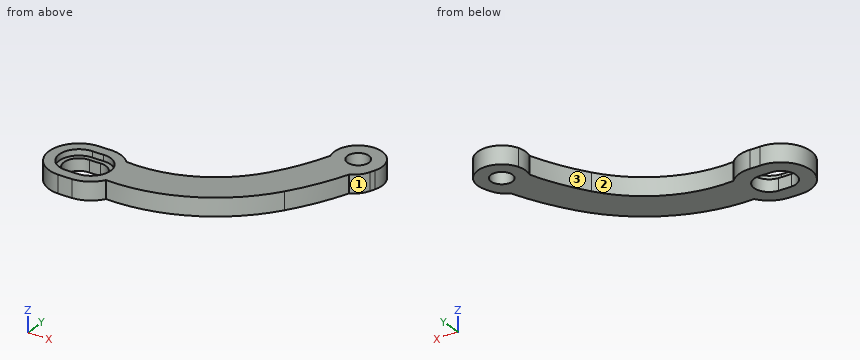
Autodesk Inventor part; units mm, degrees
ref_plane "YZ Plane" through (0, 0, 0) normal (1, 0, 0) x (0, 1, 0)
ref_plane "XZ Plane" through (0, 0, 0) normal (0, 1, 0) x (-1, 0, 0)
ref_plane "XY Plane" through (0, 0, 0) normal (0, 0, 1) x (1, 0, 0)
sketch "Sketch1" plane through (0, 0, 0) normal (0, 0, 1) x (1, 0, 0)
  circle A0 centre (31, 22) radius 1.25
  circle A1 centre (31, 22) radius 3
  arc A2 (0, 0) -> (31, 22) centre (-0.1128, 32.9998) ccw construction
  arc A3 (0.0103, -3) -> (33.8284, 21) centre (-0.1128, 32.9998) ccw
  arc A4 (-0.0103, 3) -> (28.1716, 23) centre (-0.1128, 32.9998) ccw
  arc A5 (-0.0103, 3) -> (0.0103, -3) centre (0, 0) ccw
  arc A6 (33.8284, 21) -> (28.1716, 23) centre (31, 22) ccw
  point P0 (41.5332, 21.1583)
  point P1 (35.8668, 23.1312)
  point P2 (33.8284, 21)
  point P3 (28.1716, 23)
  dimension "d1" = 30
  dimension "d21" = 6
  dimension "d22" = 2.5
  dimension "d23" = 31
  dimension "d24" = 22
extrude "Extrusion1" add sketch "Sketch1" along normal blind 3
sketch "Sketch3" plane through (0, 0, 3) normal (0, 0, 1) x (1, 0, 0)
  arc A0 (-1, 0.0117) -> (1, 0.0186) centre (-0.1128, 32.9998) ccw construction
  arc A1 (-1.1344, -4.9865) -> (1.1686, -4.9786) centre (-0.1128, 32.9998) ccw
  arc A2 (-0.8656, 5.0099) -> (0.8314, 5.0157) centre (-0.1128, 32.9998) ccw
  arc A3 (-0.8656, 5.0099) -> (-1.1344, -4.9865) centre (-1, 0.0117) ccw
  arc A4 (1.1686, -4.9786) -> (0.8314, 5.0157) centre (1, 0.0186) ccw
  arc A5 (0.0103, -3) -> (33.8284, 21) centre (-0.1128, 32.9998) ccw
  point P0 (0, 0)
  dimension "d31" = 10
  dimension "d32" = 1
  dimension "d33" = 1
extrude "Extrusion3" add sketch "Sketch3" against normal blind 3
sketch "Sketch4" plane through (0, 0, 3) normal (0, 0, -1) x (1, 0, 0)
  arc A0 (-1.1344, 4.9865) -> (-0.8656, -5.0099) centre (-1, -0.0117) ccw
  arc A1 (1.1686, 4.9786) -> (-1.1344, 4.9865) centre (-0.1128, -32.9998) ccw
  arc A2 (0.8314, -5.0157) -> (-0.8656, -5.0099) centre (-0.1128, -32.9998) ccw
  arc A3 (1, -0.0186) -> (-1, -0.0117) centre (-0.1128, -32.9998) ccw construction
  arc A4 (1.0843, 2.48) -> (-1.0672, 2.4874) centre (-0.1128, -32.9998) ccw
  arc A5 (0.9157, -2.5172) -> (-0.9328, -2.5108) centre (-0.1128, -32.9998) ccw
  arc A6 (0.9157, -2.5172) -> (1.0843, 2.48) centre (1, -0.0186) ccw
  arc A7 (-1.0672, 2.4874) -> (-0.9328, -2.5108) centre (-1, -0.0117) ccw
  arc A8 (28.1716, -23) -> (4.6946, -3.3875) centre (-0.1128, -32.9998) ccw
  arc A9 (28.1716, -23) -> (33.8284, -21) centre (31, -22) ccw
  arc A10 (33.8284, -21) -> (5.2614, 2.5968) centre (-0.1128, -32.9998) ccw
  arc A11 (5.2614, 2.5968) -> (1.1686, 4.9786) centre (1, -0.0186) ccw
  arc A12 (0.8314, -5.0157) -> (4.6946, -3.3875) centre (1, -0.0186) ccw
  arc A13 (0.8887, -3.3167) -> (-0.9113, -3.3105) centre (-0.1128, -32.9998) ccw
  arc A14 (0.8887, -3.3167) -> (1.1113, 3.2795) centre (1, -0.0186) ccw
  arc A15 (1.1113, 3.2795) -> (-1.0887, 3.2871) centre (-0.1128, -32.9998) ccw
  arc A16 (-1.0887, 3.2871) -> (-0.9113, -3.3105) centre (-1, -0.0117) ccw
  point P0 (0, 0)
  dimension "d43" = 5
  dimension "d52" = 0.8
extrude "Extrusion4" cut sketch "Sketch4" along normal through all contours A6 A5 A7 A4
sketch "Sketch5" plane through (0, 0, 3) normal (0, 0, 1) x (1, 0, 0)
  circle A0 centre (31, 22) radius 1.25
  arc A1 (0, 0) -> (31, 22) centre (-0.1128, 32.9998) ccw construction
  arc A2 (34.7535, 20.6174) -> (27.2465, 23.3826) centre (31, 22) ccw
  arc A3 (26.9479, 22.5719) -> (34.4549, 19.8068) centre (30.7014, 21.1893) ccw
  line L0 (30.0441, 21.4413) -> (31.2665, 20.9727)
  line L1 (32.5586, 21.449) -> (29.5201, 22.5232)
  line L2 (26.9479, 22.5719) -> (27.2465, 23.3826)
  line L3 (34.4549, 19.8068) -> (34.7535, 20.6174)
  circle A4 centre (31, 22) radius 1.8
  dimension "d44" = 8
  dimension "d46" = 1.5
  dimension "d47" = 3.6
extrude "Extrusion5" cut sketch "Sketch5" against normal up to surface (3 mm away) contours A4
extrude "Extrusion6" add sketch "Sketch5" against normal up to surface (3 mm away) contours L3 A3 L2 A2
extrude "Extrusion7" cut sketch "Sketch4" along normal blind 1 contours A13 A16 A15 A14
sketch "Sketch6" plane through (0, 0, 0) normal (0, 0, -1) x (-1, 0, 0)
  circle A0 centre (-31, 22) radius 1.8
  arc A1 (-32.4154, 17.5752) -> (-5.2614, -2.5968) centre (0.1128, 32.9998) ccw
  arc A2 (-5.2614, -2.5968) -> (-1.1686, -4.9786) centre (-1, 0.0186) ccw
  arc A3 (-1.1686, -4.9786) -> (1.1344, -4.9865) centre (0.1128, 32.9998) ccw
  arc A4 (1.1344, -4.9865) -> (0.8656, 5.0099) centre (1, 0.0117) ccw
  arc A5 (-0.8314, 5.0157) -> (0.8656, 5.0099) centre (0.1128, 32.9998) ccw
  arc A6 (-0.8314, 5.0157) -> (-4.6946, 3.3875) centre (-1, 0.0186) ccw
  arc A7 (-26.899, 19.9475) -> (-4.6946, 3.3875) centre (0.1128, 32.9998) ccw
  arc A8 (-26.899, 19.9475) -> (-26.9479, 22.5719) centre (-30.7014, 21.1893) ccw
  line L0 (-26.9479, 22.5719) -> (-27.2465, 23.3826)
  arc A9 (-27.2465, 23.3826) -> (-34.7535, 20.6174) centre (-31, 22) ccw
  line L1 (-34.7535, 20.6174) -> (-34.4549, 19.8068)
  arc A10 (-34.4549, 19.8068) -> (-32.4154, 17.5752) centre (-30.7014, 21.1893) ccw
  arc A11 (-1.0843, -2.48) -> (1.0672, -2.4874) centre (0.1128, 32.9998) ccw
  arc A12 (-0.9157, 2.5172) -> (-1.0843, -2.48) centre (-1, 0.0186) ccw
  arc A13 (-0.9157, 2.5172) -> (0.9328, 2.5108) centre (0.1128, 32.9998) ccw
  arc A14 (1.0672, -2.4874) -> (0.9328, 2.5108) centre (1, 0.0117) ccw
  arc A15 (-27.2465, 23.3826) -> (-34.7535, 20.6174) centre (-31, 22) ccw
  arc A16 (-27.2315, 20.6591) -> (-27.2465, 23.3826) centre (-31, 22) ccw
  arc A17 (-26.899, 19.9475) -> (-4.6946, 3.3875) centre (0.1128, 32.9998) ccw
  arc A18 (-27.2315, 20.6591) -> (-26.899, 19.9475) centre (0.1128, 32.9998) ccw
  arc A19 (-26.899, 19.9475) -> (-4.6946, 3.3875) centre (0.1128, 32.9998) ccw
  point P0 (0, 0)
extrude "Extrusion8" cut sketch "Sketch6" against normal up to surface (3 mm away) contours L0 A8 A18 A16
sketch "Sketch7" plane through (0, 0, 3) normal (0, 0, 1) x (1, 0, 0)
  arc A0 (34.7535, 20.6174) -> (27.2315, 20.6591) centre (31, 22) ccw
  arc A1 (4.6946, 3.3875) -> (27.2315, 20.6591) centre (-0.1128, 32.9998) ccw
  arc A2 (4.6946, 3.3875) -> (0.8314, 5.0157) centre (1, 0.0186) ccw
  arc A3 (-0.8656, 5.0099) -> (0.8314, 5.0157) centre (-0.1128, 32.9998) ccw
  arc A4 (-0.8656, 5.0099) -> (-1.1344, -4.9865) centre (-1, 0.0117) ccw
  arc A5 (-1.1344, -4.9865) -> (1.1686, -4.9786) centre (-0.1128, 32.9998) ccw
  arc A6 (1.1686, -4.9786) -> (5.2614, -2.5968) centre (1, 0.0186) ccw
  arc A7 (5.2614, -2.5968) -> (32.4154, 17.5752) centre (-0.1128, 32.9998) ccw
  arc A8 (32.4154, 17.5752) -> (34.4549, 19.8068) centre (30.7014, 21.1893) ccw
  line L0 (34.4549, 19.8068) -> (34.7535, 20.6174)
  circle A9 centre (31, 22) radius 1.8
  arc A10 (-1.0887, -3.2871) -> (1.1113, -3.2795) centre (-0.1128, 32.9998) ccw
  arc A11 (-0.9113, 3.3105) -> (-1.0887, -3.2871) centre (-1, 0.0117) ccw
  arc A12 (-0.9113, 3.3105) -> (0.8887, 3.3167) centre (-0.1128, 32.9998) ccw
  arc A13 (1.1113, -3.2795) -> (0.8887, 3.3167) centre (1, 0.0186) ccw
  arc A14 (5.2614, -2.5968) -> (32.4154, 17.5752) centre (-0.1128, 32.9998) ccw
  arc A15 (5.2614, -2.5968) -> (27.6993, 8.5472) centre (6.5569, 22.9556) ccw
  arc A16 (27.6993, 8.5472) -> (32.4154, 17.5752) centre (-8.4143, 33.1583) ccw
  arc A17 (4.6946, 3.3875) -> (22.8001, 11.886) centre (6.5569, 22.9556) ccw
  arc A18 (34.7535, 20.6174) -> (27.2315, 20.6591) centre (31, 22) ccw
  arc A19 (22.8001, 11.886) -> (27.2315, 20.6591) centre (-8.4143, 33.1583) ccw
  line L1 (5.2614, -2.5968) -> (4.6946, 3.3875)
  line L2 (4.6946, 3.3875) -> (2.1704, 20.8058)
  line L3 (2.1704, 20.8058) -> (15.0141, 27.6003)
  line L4 (15.0141, 27.6003) -> (27.2315, 20.6591)
  point P0 (0, 0)
extrude "Extrusion9" cut sketch "Sketch7" against normal up to surface (3 mm away) contours A19 A17 A1 | A1 L2 L3 L4
extrude "Extrusion10" add sketch "Sketch7" against normal up to surface (3 mm away) contours A16 A15 A7
Read the model definition and answer for the solid it produces. Units are mm, in the model's axes. Face numbers are marked on the shaded views. Give positions to 0.01 mm unless a question says otherwise; leave off trailing zeros. Order: outer loops, then holes, each group sorted by start corner. A loop starts at its lowest first (then second) coordinate and runs counter-clockwise, first axis right, second up.
(1) For a pull along X with two mould halves and no side action, classify the marked faces 1, 2 and 3 as released by +X, released by -X, zero draft, split by the parting line, or undercut.
(2) Given pin 1 (3.5 mm diameter, centred on x = -2, y = -0.5, fed in from +Z); pin 2 (3 mm diameter, centred on x = 31, y = 22, fed in from -Z), each flat-ended and moving along its own axis, determine where each tip first touches the part or whether it passes through.
(3) Straight lines are drawn through the part: L1, parallel to Y at x = 1, z = 0.7; L2, parallel to Y at x = 3, z = 0.75; L3, parallel to X at y = 7, z = 1.8. For each, find the intervals that lie inside material, in ascending order.
(4) Find section B-B (z = 0.5). Give the vertices of the cut face in (x, y).
(5) Find section D-D (x = 8). Give the vertices of the cut face in (y, z).
(6) Find section A-A (y = 22). Give the vertices of the cut face in (x, z).
(7) Find section C-C (y = -1). Give the vertices of the cut face in (x, z), plus the area to 3 significant figures.
Result sheet:
1. face 1: released by +X
1. face 2: undercut
1. face 3: released by -X
2. pin 1: stops at z = 2
2. pin 2: passes through
3. L1: y = -4.98 to -2.48, 2.52 to 5.02
3. L2: y = -4.56 to -1.48, 1.52 to 4.6
3. L3: x = 18.04 to 26.56
4. outline: (-1.13, -4.99) arc R37.97 ccw to (1.17, -4.98) arc R5 ccw to (5.26, -2.6) arc R25.59 ccw to (27.7, 8.55) arc R43.7 ccw to (32.42, 17.58) arc R4 ccw to (34.45, 19.81) - (34.75, 20.62) arc R4 ccw to (27.25, 23.38) arc R4 ccw to (27.23, 20.66) arc R37.78 cw to (22.8, 11.89) arc R19.66 cw to (4.69, 3.39) arc R5 ccw to (0.83, 5.02) arc R28 cw to (-0.87, 5.01) arc R5 ccw to start; hole (-1.07, -2.49) arc R35.55 ccw to (1.08, -2.48) arc R2.5 ccw to (0.92, 2.52) arc R30.59 cw to (-0.93, 2.51) arc R2.5 ccw to start; hole circle Ø3.6 at (31, 22)
5. outline: (-2.59, 0) - (3.35, 0) - (3.35, 3) - (-2.59, 3) - close
6. outline: (27, 0) - (29.2, 0) - (29.2, 3) - (27, 3) - close; (32.8, 0) - (35, 0) - (35, 3) - (32.8, 3) - close
7. outline: (-5.9, 0) - (-3.29, 0) - (-3.29, 2) - (-4.14, 2) - (-4.14, 3) - (-5.9, 3) - close; (3.28, 0) - (15.54, 0) - (15.54, 3) - (4.14, 3) - (4.14, 2) - (3.28, 2) - close
7. area: 42.9 mm2
